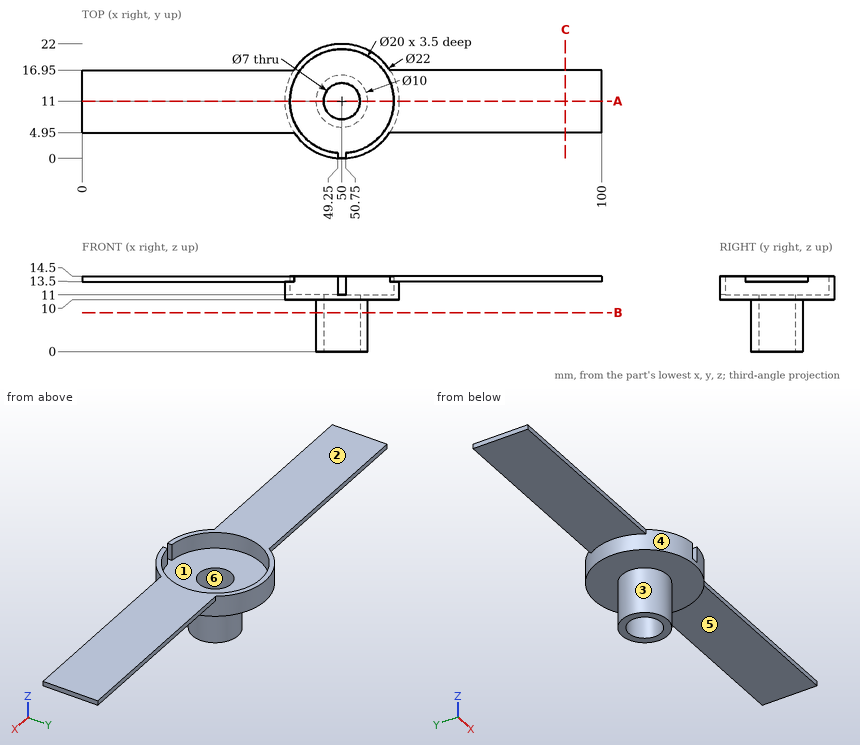
Drawing for the job (mm, zero at the part's lowest x, y, z). A direction names the side the tool comes from. Give positions to 0.01 mm unless a question says otherwise; leave off trailing zeros. Order: outer loops, then holes, each group sorted by start corner. A loop starts at its lowest first (then second) coordinate and runs counter-clockwise, first axis right, second up. Notation, with made-up numbers: (4.25, -23.5) -> (12.25, -23.5) arc R22 ccw to (12.25, 13.5) -> close; hole circle Ø3 at (-39, 13). An arc over 180 degrees is marked (long way). Use one line per item in the form item = value.
(1) Flat gauge pins, fed straight in: P1, Ø3.5, axis at x = 23, y = 8.5, coming from the -Z side; P2, Ø0.8, axis at y = 0.5, z = 12.5, coming from the +X side (1 decimal); P3, Ø8, axis at x = 50, y = 11, coming from the +Z side. Where does each tip first touch, or does it go through?
Solution:
P1 = 13.5
P2 = 54.4
P3 = 11
(2) Saw through at A-A (y = 11). Write the cut outline in (x, z).
Solution:
outline = (0, 13.5) -> (39, 13.5) -> (39, 10) -> (45, 10) -> (45, 0) -> (46.5, 0) -> (46.5, 11) -> (40, 11) -> (40, 14.5) -> (0, 14.5) -> close; (53.5, 0) -> (55, 0) -> (55, 10) -> (61, 10) -> (61, 13.5) -> (100, 13.5) -> (100, 14.5) -> (60, 14.5) -> (60, 11) -> (53.5, 11) -> close
(3) Tool access for the marked faces 1, 2 and 3: list every direction of +Z, -Z, +X, -X, +Y, -Y with a clear straight run to the whole face (end or side of a thin tool).
Solution:
face_1 = +Z
face_2 = +Z, +X, -X, +Y, -Y
face_3 = -Z
(4) Saw through at C-C (x = 93). Write the cut outline in (y, z), then the cut area to 3 significant figures.
Solution:
outline = (4.95, 13.5) -> (16.95, 13.5) -> (16.95, 14.5) -> (4.95, 14.5) -> close
area = 12.0 mm²
(5) Drill centre lines: line 1 (X direction, y = 11, z = 11.9); line 2 (Y direction, x = 50, z = 2.75); line 3 (Z direction, x = 33, y = 13.75). Where is each one in solid material? Low to high. Write a range as from..to.
Solution:
line_1 = 39..40, 60..61
line_2 = 6..7.5, 14.5..16
line_3 = 13.5..14.5
(6) Saw through at B-B (z = 7.5). Write the cut outline in (x, y).
Solution:
outline = circle Ø10 at (50, 11); hole circle Ø7 at (50, 11)
(7) Pull direction X, two halves, no side cores. Call the marked faces 4, 5 and 6: +X half, -X half, draft (parallel to the pull), parting line (faces both ways), or undercut.
Solution:
face_4 = parting line
face_5 = draft
face_6 = undercut
